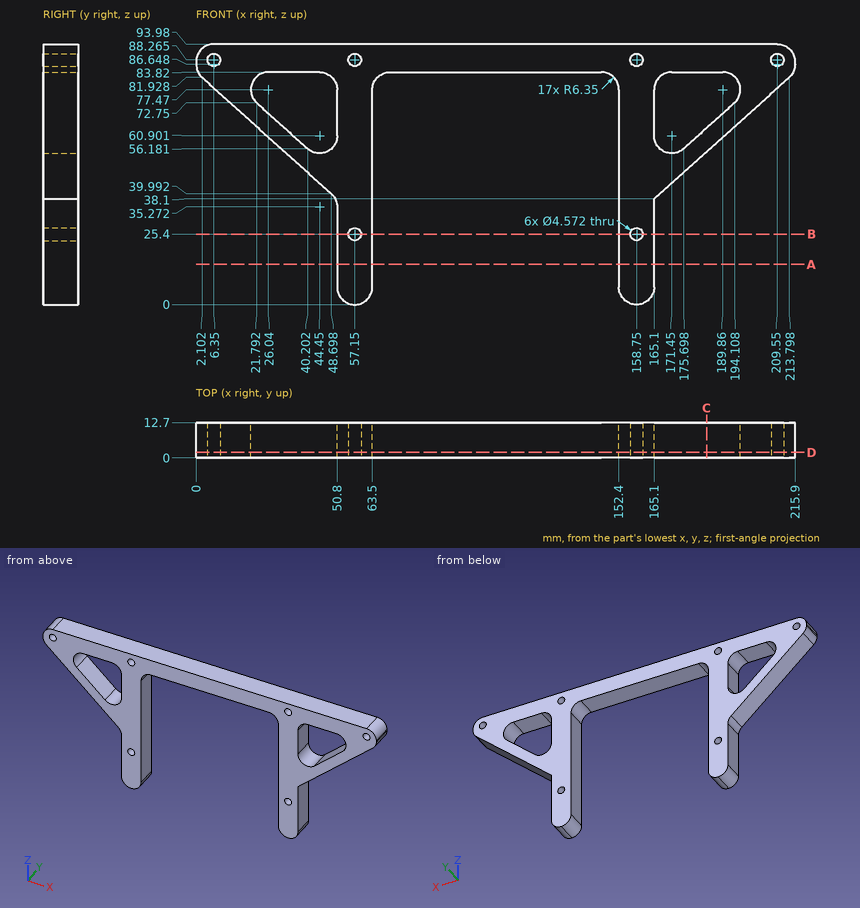
Input: dimensioned drawing with shaded views. Units: mm. Origin: part minimum x, y, z. Give positions to 0.01 mm unless a question says otherwise; leave off trailing zeros. Write each loop counter-clockwise with the first axis right and the second up, starting at its lowest first coordinate (ties: lowest second). Pieces come first, ordered by that corner, then holes. Notation, with made-up numbers: (40, -16.75) - (86, -16.75) arc R22 ccw to (86, 7.25) - close; hole circle Ø2 at (-14, 52). An arc over 180 degrees is marked (long way). One line per item, written item: value. Start each with the question number.
Q1. Section query C-C, the plane x = 184. Return the cut outline in (y, z).
Q2. First-contact query: pin 1 Ø6.5 at (x, y) = (177.5, 4) entering from -Z (1 decimal); pin 2 Ø1.5 at (y, z) = (7, 74) entering from +X; pin 3 Ø5 at (y, z) = (8.5, 28) entering from -X. Flat tips, straight axial feed; report the tip coordinate or a pass-through.
Q3. Section query D-D, the plane y = 2. Count the separate pieces of the cut face and the enclosed holes in it, then the cut area to 3 significant figures.
Q4. Section query B-B, the plane z = 25.4. Return the cut outline in (x, y).
Q5. Material intervals for probe 1 along X at (y, z) = (9.75, 25.4); probe 2 along Z at (x, y) = (158.75, 3); probe 3 along X at (y, z) = (11.5, 30), sorted ascending. Write a range as from..to.
Q6. Section query A-A, the plane z = 14.5. Return the cut outline in (x, y).
Answer:
1. outline: (0, 55.11) - (12.7, 55.11) - (12.7, 63.65) - (0, 63.65) - close; (0, 83.82) - (12.7, 83.82) - (12.7, 93.98) - (0, 93.98) - close
2. pin 1: stops at z = 46.3
2. pin 2: stops at x = 205.82
2. pin 3: stops at x = 50.8
3. separate pieces: 1
3. enclosed holes: 8
3. area: 5,190 mm2
4. outline: (50.8, 0) - (54.86, 0) - (54.86, 12.7) - (50.8, 12.7) - close; (59.44, 0) - (63.5, 0) - (63.5, 12.7) - (59.44, 12.7) - close; (152.4, 0) - (156.46, 0) - (156.46, 12.7) - (152.4, 12.7) - close; (161.04, 0) - (165.1, 0) - (165.1, 12.7) - (161.04, 12.7) - close
5. probe 1: x = 50.8..54.86, 59.44..63.5, 152.4..156.46, 161.04..165.1
5. probe 2: z = 0..23.11, 27.69..85.98, 90.55..93.98
5. probe 3: x = 50.8..63.5, 152.4..165.1
6. outline: (50.8, 0) - (63.5, 0) - (63.5, 12.7) - (50.8, 12.7) - close; (152.4, 0) - (165.1, 0) - (165.1, 12.7) - (152.4, 12.7) - close
